Could you check a few things on this drawing? It's one solid part, dimensions in mm from its lowest x, y, z. Round coordinates to 2 decimals unless told otherwise and drop trailing zeros. Write each loop counter-clockwise with the first axis right and the second up, starting at its lowest first coordinate (ties: lowest second). Pieces come first, ordered by that corner, then holes. Notation, with made-up numbers: (3, 64) - (45, 64) arc R25 cw to (45, 87) - close; hole circle Ø9 at (24, 87). An arc over 180 degrees is marked (long way). Put each result on its own line as item: value.
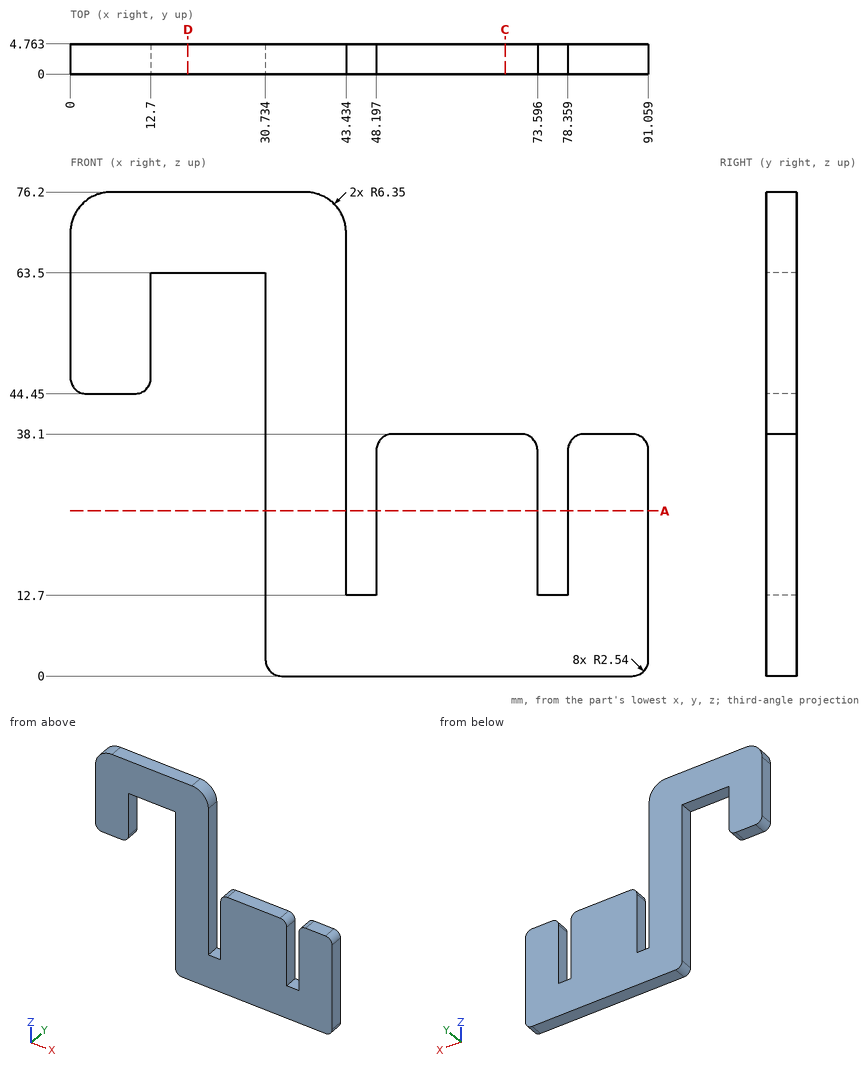
(1) Imagine slicing it at A-A, the plane z = 26. List the corners of the cut face in (x, y) for me (1 decimal), then the cut area to 3 significant figures.
Values found:
outline: (30.7, 0) - (43.4, 0) - (43.4, 4.8) - (30.7, 4.8) - close; (48.2, 0) - (73.6, 0) - (73.6, 4.8) - (48.2, 4.8) - close; (78.4, 0) - (91.1, 0) - (91.1, 4.8) - (78.4, 4.8) - close
area: 242 mm^2
(2) Imagine slicing it at D-D, the plane x = 18.5. List the corners of the cut face in (y, z) for me.
Values found:
outline: (0, 63.5) - (4.76, 63.5) - (4.76, 76.2) - (0, 76.2) - close
(3) Please list where these lines run through material, in increasing order: probe 1 along X at (y, z) = (2.9, 27) (1 decimal); probe 2 along X at (y, z) = (2.4, 62.5) (1 decimal); probe 3 along Z at (x, y) = (58.5, 1.05). Write a range as from..to.
Values found:
probe 1: x = 30.7..43.4, 48.2..73.6, 78.4..91.1
probe 2: x = 0..12.7, 30.7..43.4
probe 3: z = 0..38.1
(4) I'm going to push flat-ended pins straight in: pin 1 (1 mm diameter, centred on y = 0.5, z = 50, fed in from +X); pin 2 (1.4 mm diameter, centred on x = 26, y = 3, fed in from -Z). Where does each tip first touch, or does it pass through?
Values found:
pin 1: stops at x = 43.43
pin 2: stops at z = 63.5
(5) Imagine slicing it at C-C, the plane x = 68.5. List the corners of the cut face in (y, z) for me.
Values found:
outline: (0, 0) - (4.76, 0) - (4.76, 38.1) - (0, 38.1) - close
